from build123d import *

# Parameters (mm, degrees)
BOSS_EXTRUDE1_DEPTH = 2
SKETCH2_W           = 74
SKETCH2_H           = 2
BOSS_EXTRUDE2_DEPTH = 23
FILLET1_R           = 2
SKETCH3_R           = 5
SKETCH3_R_2         = 1.5
CUT_EXTRUDE1_DEPTH  = 26
SKETCH5_R           = 1.5
CUT_EXTRUDE2_DEPTH  = 46


with BuildPart() as part:
    # Sketch1 → Boss-Extrude1 (new body)
    with BuildSketch(Plane(origin=(0, 0, 0), x_dir=(0, 0, -1), z_dir=(1, 0, 0))):
        with BuildLine():
            Line((-14.5, 45), (14.5, 45))
            ThreePointArc((14.5, 45), (30.409902577, 38.409902577), (37, 22.5))
            Line((37, 22.5), (37, 0))
            Line((37, 0), (-37, 0))
            Line((-37, 0), (-37, 22.5))
            ThreePointArc((-37, 22.5), (-30.409902577, 38.409902577), (-14.5, 45))
        make_face()
    extrude(amount=BOSS_EXTRUDE1_DEPTH)

    # Sketch2 → Boss-Extrude2 (add)
    with BuildSketch(Plane.ZY):
        with Locations((0, 1)):
            Rectangle(SKETCH2_W, SKETCH2_H)
    extrude(amount=BOSS_EXTRUDE2_DEPTH)

    # Fillet1
    fillet1_edges = [part.edges().sort_by_distance(p)[0] for p in [
        (2, 0, 0),
        (0, 2, 0),
    ]]
    fillet(fillet1_edges, radius=FILLET1_R)

    # Sketch3 → Cut-Extrude1 (cut, through all)
    with BuildSketch(Plane(origin=(2, 0, 0), x_dir=(0, 0, -1), z_dir=(1, 0, 0))):
        with Locations((0, 30.5)):
            Circle(SKETCH3_R)
        with Locations((6.25, 35.825317547)):
            Circle(SKETCH3_R_2)
        with Locations((6.25, 14.174682453)):
            Circle(SKETCH3_R_2)
        with Locations((-12.5, 25)):
            Circle(SKETCH3_R_2)
    extrude(amount=-CUT_EXTRUDE1_DEPTH, mode=Mode.SUBTRACT)

    # Sketch5 → Cut-Extrude2 (cut, through all)
    with BuildSketch(Plane.XZ):
        with Locations((-16, -30)):
            Circle(SKETCH5_R)
        with Locations((-5, -30)):
            Circle(SKETCH5_R)
        with Locations((-5, 30)):
            Circle(SKETCH5_R)
        with Locations((-16, 30)):
            Circle(SKETCH5_R)
    extrude(amount=-CUT_EXTRUDE2_DEPTH, mode=Mode.SUBTRACT)


solid = part.part
Source: CAD feature listing. Evaluate the final solid. Frame: model axes, mm. A direction names the side the tool comes from. Coordinates: 2 decimals unless noted, no trailing zeros. Write each loop counter-clockwise with the first axis right and the second up, starting at its lowest first coordinate (ties: lowest second). Pieces come first, ordered by that corner, then holes. Notation, with made-up numbers: M -8.5,81 L 24.5,81 A11 cw 24.5,92 Z; hole C 21.25,19 d2. An arc over 180 degrees is marked long. Use a Markdown table: item, result.
1) Ray query, L1, parallel to Z at x = -5, y = 0.8; L2, parallel to X at y = 41, z = 1.5. Return the intervals inside material, ascending.
Conclusion:
| item | result |
|---|---|
| L1 | z = -37 to -31.5, -28.5 to 28.5, 31.5 to 37 |
| L2 | x = 0 to 2 |
2) Reachability of faces 1 (the cylindrical face through (1.4, 0.57, 0.52)), 2 (the flat face through (-12, 2, -1)) from +Z, -Z, +X, -X, +Y, -Y: full face, straight path, thin tool, end or side. Return the list, or none.
Conclusion:
| item | result |
|---|---|
| face 1 | +Z, -Z, +X, -Y |
| face 2 | +Z, -Z, -X, +Y |
3) First-contact query: pin 1 Ø1.8 at (x, z) = (-5, 30) entering from +Y; pin 2 Ø5 at (y, z) = (36, 7) entering from -X; pin 3 Ø10.5 at (x, z) = (-10, 1) entering from +Y. Flat tips, straight axial feed; report the tip coordinate or a pass-through.
Conclusion:
| item | result |
|---|---|
| pin 1 | passes through |
| pin 2 | stops at x = 0 |
| pin 3 | stops at y = 2 |
4) Section C-C, the plane z = 30. Output: boundary loops of the cut face in (x, y).
Conclusion:
| item | result |
|---|---|
| outline | M -23,0 L -17.5,0 L -17.5,2 L -23,2 Z; M -14.5,0 L -6.5,0 L -6.5,2 L -14.5,2 Z; M -3.5,0 L 0,0 A2 ccw 2,2 L 2,38.81 L 0,38.81 L 0,4 A2 cw -2,2 L -3.5,2 Z |
5) Mould query, pull axis Y, two halves, no side actions, for faces 3 (the flat face through (2, 24, -1)), 4 (the cylindrical face through (-0.57, 2.6, 0.52)), 5 (the cylindrical face through (1.01, 15.66, -6.05)), 6 (the cylindrical face through (1.014, 26.487, 12.695)). Classes: pulls with the +Y half, pulls with the -Y half, needs draft (parallel to the pull), parting line crosses it, or undercut.
Conclusion:
| item | result |
|---|---|
| face 3 | needs draft |
| face 4 | pulls with the +Y half |
| face 5 | undercut |
| face 6 | undercut |
6) Section D-D, the plane x = -11.75. Output: boundary loops of the cut face in (y, z), then the cut area to 3 significant figures.
Conclusion:
| item | result |
|---|---|
| outline | M 0,-37 L 2,-37 L 2,37 L 0,37 Z |
| area | 148 mm^2 |
7) Section B-B, the plane x = -16. Output: boundary loops of the cut face in (y, z), then the cut area to 3 significant figures.
Conclusion:
| item | result |
|---|---|
| outline | M 0,-37 L 2,-37 L 2,-31.5 L 0,-31.5 Z; M 0,-28.5 L 2,-28.5 L 2,28.5 L 0,28.5 Z; M 0,31.5 L 2,31.5 L 2,37 L 0,37 Z |
| area | 136 mm^2 |
8) Section A-A, the plane z = 0. Output: boundary loops of the cut face in (x, y).
Conclusion:
| item | result |
|---|---|
| outline | M -23,0 L 0,0 A2 ccw 2,2 L 2,25.5 L 0,25.5 L 0,4 A2 cw -2,2 L -23,2 Z; M 0,35.5 L 2,35.5 L 2,45 L 0,45 Z |
